```python
from build123d import *

# Parameters (mm, degrees)
SKETCH2_R          = 5
CUT_EXTRUDE1_DEPTH = 66.421885576
SKETCH3_R          = 10
CUT_EXTRUDE2_DEPTH = 71.540932177


with BuildPart() as part:
    # Sketch1 → Revolve1 (revolve)
    with BuildSketch(Plane(origin=(0, 0, 0), x_dir=(1, 0, 0), z_dir=(0, 1, 0)), mode=Mode.PRIVATE) as revolve1_sk:
        Polygon((0, 0), (0, 16), (12, 18), (12, 35), (0, 38), (0, 43.307176728), (35, 43.307176728), (35, 38), (23, 35), (23, 18), (35, 16), (35, 0), align=None)
    revolve(revolve1_sk.sketch.rotate(Axis((0, 0, 0), (1, 0, 0)), 180), axis=Axis((0, 0, 0), (1, 0, 0)))

    # Sketch2 → Cut-Extrude1 (cut, through all)
    with BuildSketch(Plane(origin=(23, 0, 0), x_dir=(0, 0, -1), z_dir=(1, 0, 0))):
        with Locations((0, 28)):
            Circle(SKETCH2_R)
        with Locations((28, 0)):
            Circle(SKETCH2_R)
        with Locations((0, -28)):
            Circle(SKETCH2_R)
        with Locations((-28, 0)):
            Circle(SKETCH2_R)
    extrude(amount=-CUT_EXTRUDE1_DEPTH, mode=Mode.SUBTRACT)

    # Sketch3 → Cut-Extrude2 (cut, through all)
    with BuildSketch(Plane(origin=(35, 0, 0), x_dir=(0, 0, -1), z_dir=(1, 0, 0))):
        Circle(SKETCH3_R)
    extrude(amount=-CUT_EXTRUDE2_DEPTH, mode=Mode.SUBTRACT)


solid = part.part
```
Part model, mm, in its own coordinate system. A direction names the side the tool comes from. Round coordinates to 2 decimals unless told otherwise and drop trailing zeros. Order: outer loops, then holes, each group sorted by start corner. A loop starts at its lowest first (then second) coordinate and runs counter-clockwise, first axis right, second up. Notation, with made-up numbers: M 50.5,30.5 L 104.5,30.5 A27 cw 104.5,67.5 Z; hole C 28.25,37 d10. An arc over 180 degrees is marked long. Answer in a Markdown table with one row per item. Add a question column.
Q1. Cut at C-C on x = 18.5. Give the cut face in (y, z).
Q2. Cut at B-B on x = 9.5. Give the cut face in (y, z) (3 decimals), and give its area (3 significant figures).
Q3. Pin check, flat tips, straight feed: pin 1 (10 mm diameter, centred on x = 14.5, y = -11.5, fed in from -Z); pin 2 (2 mm diameter, centred on x = 18.5, z = -12.5, fed in from -Y); pin 3 (3 mm diameter, centred on x = 24, z = -17.5, fed in from -Y); pin 4 (16 mm diameter, centred on y = 0, z = 0, fed in from +X). Stop position of each tip, or through.
Q4. Cut at A-A on z = 0. Give the number of separate pieces and of enclosed holes in the cut face, and give its area (3 significant figures).
Q5. Cut at D-D on x = 28.5. Give the cut face in (y, z) (3 decimals).
Q6. Wall check: L1, parallel to Z at x = 31, y = 12.5; L2, parallel to Y at x = 15.75, z = 0; L3, parallel to Z at x = 32.5, y = 11. Give the ranges that are in metal, low to high. Write a range as from..to.
Q7. 3-axis set-ups, long thin cutter, end or side, ignore diameter. For faces 4 (the face through (0, 10.4, 0.2)), 5 (the face through (23, 15, 15)), 6 (the face through (12, 15, -15)): which of +Z, -Z, +X, -X, +Y, -Y reach the whole face in a straight line?
Q8. Mould opens along Y. For faces 1 (the face through (35, 38.3, -0.2)), 2 (the face through (18, 0, -23)), 3 (the face through (17.74, 26.35, -34.37)) say: +Y half, -Y half, draft (parallel to the pull), parting line (faces both ways), or undercut.
Established:
| question | item | result |
|---|---|---|
| 1 | outline | C 0,0 d86.61; hole C -28,0 d10; hole C 0,0 d20; hole C 0,-28 d10; hole C 0,28 d10; hole C 28,0 d10 |
| 2 | outline | C 0,0 d86.614; C 0,0 d35.167; hole C 0,0 d71.25; hole C 0,0 d20 |
| 2 | area | 2,560 mm2 |
| 3 | pin 1 | stops at z = -42.82 |
| 3 | pin 2 | stops at y = -41.75 |
| 3 | pin 3 | stops at y = -40.24 |
| 3 | pin 4 | passes through |
| 4 | separate pieces | 4 |
| 4 | enclosed holes | 0 |
| 4 | area | 1,180 mm2 |
| 5 | outline | C 0,0 d86.614; C 0,0 d34.167; hole C 0,0 d72.75; hole C 0,0 d20 |
| 6 | L1 | z = -41.46..-34.82, -11.02..11.02, 34.82..41.46 |
| 6 | L2 | y = -43.31..-33, -23..-10, 10..23, 33..43.31 |
| 6 | L3 | z = -41.89..-35.72, -12.19..12.19, 35.72..41.89 |
| 7 | face 4 | +Z, -Z, -X, +Y, -Y |
| 7 | face 5 | +X |
| 7 | face 6 | -X |
| 8 | face 1 | draft |
| 8 | face 2 | undercut |
| 8 | face 3 | parting line |
